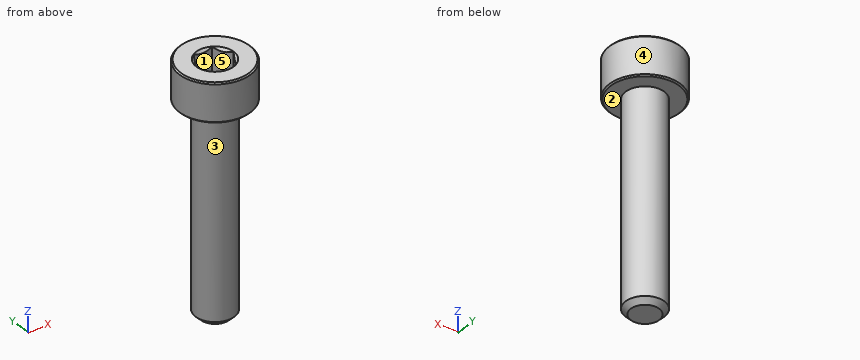
```python
from build123d import *

# Parameters (mm, degrees)
SKETCH001_R     = 3.75
POCKET_DEPTH    = 9.70192
CHAMFER_SIZE    = 0.4
CHAMFER001_SIZE = 0.1


with BuildPart() as pocket:
    # Sketch003 → Revolution001 (revolve)
    with BuildSketch(Plane.XZ):
        Polygon((0, 0.29908), (2.75, 1.3), (2.75, 10), (0, 10), align=None)
    revolve(axis=Axis((0, 0, 0), (0, 0, 1)))

    # Sketch001 → Pocket (cut, through all)
    with BuildSketch(Plane(origin=(0, 0, 10), x_dir=(-1, 0, 0), z_dir=(0, 0, 1))):
        Circle(SKETCH001_R)
        Polygon((-0.721688, 1.25), (0.721688, 1.25), (1.443376, 0), (0.721688, -1.25), (-0.721688, -1.25), (-1.443376, 0), align=None, mode=Mode.SUBTRACT)
    extrude(amount=-POCKET_DEPTH, mode=Mode.SUBTRACT)


with BuildPart() as chamfer001:
    # Sketch → Revolution (revolve)
    with BuildSketch(Plane.XZ):
        Polygon((1.45, 3), (2.75, 3), (2.75, 0), (1.5, 0), (1.5, -16), (0, -16), (0, 1.549999), align=None)
    revolve(axis=Axis((0, 0, 0), (0, 0, 1)))

    # Cut: cut Pocket
    add(pocket.part, mode=Mode.SUBTRACT)

    # Chamfer
    chamfer_edges = [chamfer001.edges().sort_by_distance(p)[0] for p in [
        (-1.5, 0, -16),
    ]]
    chamfer(chamfer_edges, length=CHAMFER_SIZE)

    # Chamfer001
    chamfer001_edges = [chamfer001.edges().sort_by_distance(p)[0] for p in [
        (-2.75, 0, 0),
        (-2.75, 0, 3),
    ]]
    chamfer(chamfer001_edges, length=CHAMFER001_SIZE)


solid = chamfer001.part
```
CAD build for the part. Positions are in the model's coordinates, mm. Face numbers are marked on the shaded views. A direction names the side the tool comes from. Round coordinates to 2 decimals unless told otherwise and drop trailing zeros. Write each loop counter-clockwise with the first axis right and the second up, starting at its lowest first coordinate (ties: lowest second). Pieces come first, ordered by that corner, then holes. Notation, with made-up numbers: (-28, -18) - (-14, -18) arc R30 ccw to (-14, 19) - close; hole circle Ø6 at (-18, 89.5). An arc over 180 degrees is marked (long way). Return JSON: item names as keys, results as strings. Group by question number.
Item 1: 3-axis set-ups, long thin cutter, end or side, ignore diameter. For the marked faces 4 and 5: which of +Z, -Z, +X, -X, +Y, -Y reach the whole face in a straight line?
Item 2: Mould opens along Y. For the marked faces 1, 2 and 3 say: +Y half, -Y half, draft (parallel to the pull), parting line (faces both ways), or undercut.
Item 3: Flat gauge pins, fed straight in: pin 1 Ø1.2 at (x, z) = (-0.5, 2) entering from +Y; pin 2 Ø1.5 at (x, z) = (2, -4.5) entering from +Y; pin 3 Ø1 at (x, z) = (-1.5, -5.5) entering from +Y. Where does each tip first touch, or does it go through?
Item 4: Probe probe 1 along Z at (x, y) = (2.35, -0.8); probe 2 along X at (y, z) = (-1.3, -6.5); probe 3 along Y at (x, z) = (1.3, 2.25). List the from-to ranges inside material, lowest first.
Item 5: Band-saw the part on A-A on z = -10.5. List the corners of the cut face in (x, y).
Resolved:
{
 "1": {"face 4": "+Z, -Z", "face 5": "+Z"},
 "2": {"face 1": "undercut", "face 2": "draft", "face 3": "parting line"},
 "3": {"pin 1": "stops at y = 2.75", "pin 2": "stops at y = 0.83", "pin 3": "stops at y = 1.12"},
 "4": {"probe 1": "z = 0 to 3", "probe 2": "x = -0.75 to 0.75", "probe 3": "y = -2.42 to -0.25, 0.25 to 2.42"},
 "5": {"outline": "circle Ø3 at (0, 0)"}
}
